Verification items for the finished model (mm, model axes). A direction names the side the tool comes from. Coordinates: 2 decimals unless noted, no trailing zeros. Loops run counter-clockwise (first coordinate to the right, second up) from the corner with the lowest first, then second, coordinate; pieces in that order, holes last. Notation, with made-up numbers: (2, -8) - (8, -8) arc R14 ccw to (8, 12) - close; hole circle Ø8 at (79, -21). An arc over 180 degrees is marked (long way). One line per item, written item: value. Start each with the question number.
(1) Set-up check for faces 4 (the face through (0, 7, 2.921)), 5 (the face through (2.5, 11.963, 1.4)), 6 (the face through (-2.5, 2.362, 1.4)): record each of +Z, -Z, +X, -X, +Y, -Y from which the full face is reachable in a straight line by a thin tool's end or side.
(2) Thickness scan on probe 1 along Y at (x, z) = (2.25, 0.6); probe 2 along X at (y, z) = (7.25, 1.1). Record the ranges inside material, lowest first. Write a range as [from, to].
(3) Section check A-A (x = 2.5). Record the boundary of the cut face in (y, z).
(4) Draft check along Y on faces 1 (the face through (0, 16.688, 1)), 2 (the face through (-2.5, 11.963, 1.4)), 3 (the face through (3.15, 0, 1)). Enter one of: +Y half, -Y half, draft (parallel to the pull), parting line (faces both ways), or undercut.
(5) Gauge pin test, flat ends, axial feed: P1, Ø1, axis at y = 10, z = 2, coming from the +X side; P2, Ø0.9, axis at y = 8, z = 1, coming from the -X side; P3, Ø1, axis at x = 0.5, y = 9, coming from the -Z side. Record the tip position at first contact, or that the pin passes through.
(6) Section check B-B (z = 1.3). Record the boundary of the cut face in (x, y).
(7) Section check C-C (y = 5.75). Record the boundary of the cut face in (x, z).
```python
from build123d import *

# Parameters (mm, degrees)
F0_W     = 1.8796
F0_H     = 4.8006
F1_DEPTH = 2.921


with BuildPart() as f1:
    # F0 (on Top) → F1 (new body)
    with BuildSketch(Plane.XY):
        Polygon((3.1496, -2.3622), (3.1496, 2.3622), (1.8796, 2.3622), (0, 2.3622), (-1.8796, 2.3622), (-3.1496, 2.3622), (-3.1496, -2.3622), align=None)
        with Locations((0.9398, 4.7625)):
            Rectangle(F0_W, F0_H)
        with Locations((-0.9398, 4.7625)):
            Rectangle(F0_W, F0_H)
    extrude(amount=F1_DEPTH)

    # F2: F1 across face


with BuildPart() as f1_1:
    add(f1.part)
    add(f1.part.mirror(Plane(origin=(0, 7.1628, 1.4605), x_dir=(-1, 0, 0), z_dir=(0, 1, 0))))


solid = f1_1.part
```
Responses:
1. face 4: +Z, +X, -X, +Y, -Y
1. face 5: +Z, -Z, +X
1. face 6: +Z, -Z, -X
2. probe 1: y = [-2.36, 2.36], [11.96, 16.69]
2. probe 2: x = [-1.88, 1.88]
3. outline: (-2.36, 0) - (2.36, 0) - (2.36, 2.92) - (-2.36, 2.92) - close; (11.96, 0) - (16.69, 0) - (16.69, 2.92) - (11.96, 2.92) - close
4. face 1: +Y half
4. face 2: undercut
4. face 3: draft
5. P1: stops at x = 1.88
5. P2: stops at x = -1.88
5. P3: stops at z = 0
6. outline: (-3.15, -2.36) - (3.15, -2.36) - (3.15, 2.36) - (1.88, 2.36) - (1.88, 11.96) - (3.15, 11.96) - (3.15, 16.69) - (-3.15, 16.69) - (-3.15, 11.96) - (-1.88, 11.96) - (-1.88, 2.36) - (-3.15, 2.36) - close
7. outline: (-1.88, 0) - (1.88, 0) - (1.88, 2.92) - (-1.88, 2.92) - close
